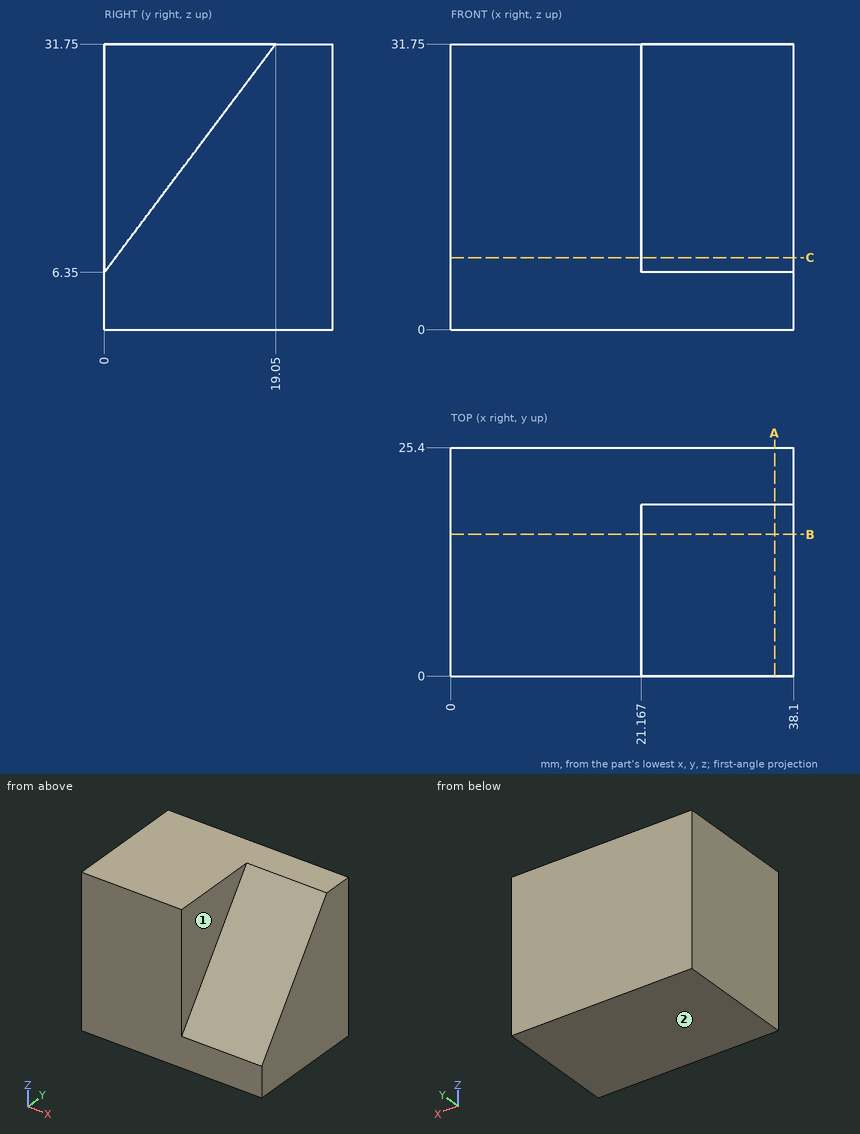
Check sheet for the drawn part. Datum: minimum x, y, z corner. Units: mm. A direction names the side the tool comes from. Round coordinates to 2 decimals unless told otherwise and drop trailing zeros. Loops run counter-clockwise (first coordinate to the right, second up) from the corner with the lowest first, then second, coordinate; pieces in that order, holes last. Notation, with made-up numbers: (33, 12) - (55, 12) arc R21 cw to (55, 17) - close; hole circle Ø3 at (-22, 89). An arc over 180 degrees is marked (long way). Answer as a JSON object with one key per item and string values. Group by question number.
Q1. Scan lines: line 1 along X through (y, z) = (7.5, 20.5); line 2 along Z through (x, y) = (32, 8) (1 decimal); line 3 along Y through (x, z) = (26, 10). Record each from-to range of solid material in increasing order. Write a range as [from, to].
Q2. Sectioned sample at A-A, the plane x = 36. Enter the section's corners in (y, z).
Q3. Sectioned sample at B-B, the plane y = 15.75. Enter the section's corners in (x, z).
Q4. Sectioned sample at C-C, the plane z = 8. Enter the section's corners in (x, y).
Q5. Set-up check for the marked faces 1 and 2: record each of +Z, -Z, +X, -X, +Y, -Y from which the full face is reachable in a straight line by a thin tool's end or side.
Solution:
{
 "1": {"line 1": "x = [0, 21.17]", "line 2": "z = [0, 17]", "line 3": "y = [2.74, 25.4]"},
 "2": {"outline": "(0, 0) - (25.4, 0) - (25.4, 31.75) - (19.05, 31.75) - (0, 6.35) - close"},
 "3": {"outline": "(0, 0) - (38.1, 0) - (38.1, 27.35) - (21.17, 27.35) - (21.17, 31.75) - (0, 31.75) - close"},
 "4": {"outline": "(0, 0) - (21.17, 0) - (21.17, 1.24) - (38.1, 1.24) - (38.1, 25.4) - (0, 25.4) - close"},
 "5": {"face 1": "+Z, +X, -Y", "face 2": "-Z, +X, -X, +Y, -Y"}
}
